from build123d import *

# Parameters (mm, degrees)
F0_W     = 19.05
F0_H     = 38.1
F1_DEPTH = 19.05
F2_W     = 19.05
F2_H     = 19.05
F3_DEPTH = 19.05
F4_W     = 19.05
F4_H     = 19.05
F5_DEPTH = 19.05
F6_W     = 19.05
F6_H     = 19.05
F7_DEPTH = 19.05


with BuildPart() as f1:
    # F0 (on Front) → F1 (new body)
    with BuildSketch(Plane.XZ):
        with Locations((-2.74175, 14.235811)):
            Rectangle(F0_W, F0_H)
    extrude(amount=F1_DEPTH)

    # F2 (on face) → F3 (join)
    with BuildSketch(Plane.XZ.offset(19.05)):
        with Locations((-2.74175, 4.710811)):
            Rectangle(F2_W, F2_H)
    extrude(amount=F3_DEPTH)

    # F4 (on face) → F5 (join)
    with BuildSketch(Plane(origin=(0, 0, -4.814189), x_dir=(1, 0, 0), z_dir=(0, 0, -1))):
        with Locations((-2.74175, 28.575)):
            Rectangle(F4_W, F4_H)
    extrude(amount=F5_DEPTH)

    # F6 (on face) → F7 (join)
    with BuildSketch(Plane.XZ.offset(38.1)):
        with Locations((-2.74175, -14.339189)):
            Rectangle(F6_W, F6_H)
    extrude(amount=F7_DEPTH)


solid = f1.part
Could you check a few things on this model? Use its own coordinates, in mm. A direction names the side the tool comes from. Coordinates: 2 decimals unless noted, no trailing zeros. Order: outer loops, then holes, each group sorted by start corner. A loop starts at its lowest first (then second) coordinate and runs counter-clockwise, first axis right, second up. Notation, with made-up numbers: (65.5, 76) -> (115.5, 76) arc R23 ccw to (115.5, 113) -> close; hole circle Ø1 at (38.25, 18). An arc over 180 degrees is marked (long way). One line per item, written item: value. Start each with the question number.
1) I'm going to push flat-ended pins straight in: pin 1 (2 mm diameter, centred on x = -0.5, z = -4, fed in from +Y); pin 2 (9.5 mm diameter, centred on x = 0.5, y = -45, fed in from +Z); pin 3 (4 mm diameter, centred on x = -6.5, z = -1.5, fed in from -Y); pin 4 (1.5 mm diameter, centred on x = -7, y = -16.5, fed in from -Z). Where does each tip first touch, or does it pass through?
2) Imagine slicing it at C-C on z = 9. List the corners of the cut face in (x, y) for me.
3) Which directions (+Z, -Z, +X, -X, +Y, -Y) give clear straight access to the entire face, cutting with the end or side of a thin tool? Please do faces 1 (the flat face through (-3, -47, -4.814)), 2 (the flat face through (-12.267, -22, -2)), 3 (the flat face through (-3, -9, -4.814)).
4) If I drill on L1, parallel to Y at x = -2.75, z = 25.5; L2, parallel to Y at x = -9.5, z = -5.5; L3, parallel to Z at x = -9.5, y = -44.5, over which ranges is the centre line in solid material (lowest first)? Write a range as [from, to].
5) Imagine slicing it at A-A on x = -6.5. List the corners of the cut face in (y, z) for me, plus the area to 3 significant figures.
6) Imagine slicing it at B-B on y = -33. List the corners of the cut face in (x, z) for me.
Answer list:
1. pin 1: stops at y = 0
1. pin 2: stops at z = -4.81
1. pin 3: stops at y = -38.1
1. pin 4: stops at z = -4.81
2. outline: (-12.27, -38.1) -> (6.78, -38.1) -> (6.78, 0) -> (-12.27, 0) -> close
3. face 1: +Z, +X, -X, -Y
3. face 2: +Z, -Z, -X, +Y, -Y
3. face 3: -Z, +X, -X, +Y
4. L1: y = [-19.05, 0]
4. L2: y = [-57.15, -19.05]
4. L3: z = [-23.86, -4.81]
5. outline: (-57.15, -23.86) -> (-19.05, -23.86) -> (-19.05, -4.81) -> (0, -4.81) -> (0, 33.29) -> (-19.05, 33.29) -> (-19.05, 14.24) -> (-38.1, 14.24) -> (-38.1, -4.81) -> (-57.15, -4.81) -> close
5. area: 1,810 mm2
6. outline: (-12.27, -23.86) -> (6.78, -23.86) -> (6.78, 14.24) -> (-12.27, 14.24) -> close
